```python
from build123d import *

# Parameters (mm, degrees)
SKETCH1_R           = 26
BOSS_EXTRUDE1_DEPTH = 14.2
SKETCH4_R           = 2.9
BOSS_EXTRUDE2_DEPTH = 12.7
SKETCH8_R           = 26
BOSS_EXTRUDE3_DEPTH = 25
SKETCH9_R           = 28.075
BOSS_EXTRUDE4_DEPTH = 17.2
SKETCH10_R          = 3.325
BOSS_EXTRUDE5_DEPTH = 16.45


with BuildPart() as part:
    # Sketch1 → Boss-Extrude1 (new body)
    with BuildSketch(Plane(origin=(0, 0, 0), x_dir=(1, 0, 0), z_dir=(0, 1, 0))):
        Circle(SKETCH1_R)
    extrude(amount=BOSS_EXTRUDE1_DEPTH)

    # Sketch4 → Boss-Extrude2 (add)
    with BuildSketch(Plane.XZ):
        with BuildLine():
            Line((27.12908409, -11.679561866), (37.990088974, -4.433027686))
            ThreePointArc((37.990088974, -4.433027686), (40.05, 0), (37.990088974, 4.433027686))
            Line((37.990088974, 4.433027686), (27.12908409, 11.679561866))
            ThreePointArc((27.12908409, 11.679561866), (22.194049101, 15.251075575), (17.545087541, 19.18775399))
            ThreePointArc((17.545087541, 19.18775399), (0, 26), (-17.545087541, 19.18775399))
            ThreePointArc((-17.545087541, 19.18775399), (-22.194049101, 15.251075575), (-27.12908409, 11.679561866))
            Line((-27.12908409, 11.679561866), (-37.990088974, 4.433027686))
            ThreePointArc((-37.990088974, 4.433027686), (-40.05, 0), (-37.990088974, -4.433027686))
            Line((-37.990088974, -4.433027686), (-27.12908409, -11.679561866))
            ThreePointArc((-27.12908409, -11.679561866), (-22.194049101, -15.251075575), (-17.545087541, -19.18775399))
            ThreePointArc((-17.545087541, -19.18775399), (0, -26), (17.545087541, -19.18775399))
            ThreePointArc((17.545087541, -19.18775399), (22.194049101, -15.251075575), (27.12908409, -11.679561866))
        make_face()
        with Locations((34.25, 0)):
            Circle(SKETCH4_R, mode=Mode.SUBTRACT)
        with Locations((-34.25, 0)):
            Circle(SKETCH4_R, mode=Mode.SUBTRACT)
    extrude(amount=-BOSS_EXTRUDE2_DEPTH)

    # Sketch8 → Boss-Extrude3 (add)
    with BuildSketch(Plane(origin=(0, 14.2, 0), x_dir=(1, 0, 0), z_dir=(0, 1, 0))):
        Circle(SKETCH8_R)
    extrude(amount=BOSS_EXTRUDE3_DEPTH)

    # Sketch9 → Boss-Extrude4 (add)
    with BuildSketch(Plane(origin=(0, 39.2, 0), x_dir=(1, 0, 0), z_dir=(0, 1, 0))):
        Circle(SKETCH9_R)
    extrude(amount=BOSS_EXTRUDE4_DEPTH)

    # Sketch10 → Boss-Extrude5 (add)
    with BuildSketch(Plane(origin=(0, 56.4, 0), x_dir=(1, 0, 0), z_dir=(0, 1, 0))):
        with Locations((13.3, 0)):
            Circle(SKETCH10_R)
        with Locations((-13.3, 0)):
            Circle(SKETCH10_R)
    extrude(amount=BOSS_EXTRUDE5_DEPTH)


solid = part.part
```
Here's how the part is built. I have some questions about the finished solid (model axes, mm). A direction names the side the tool comes from. Round coordinates to 2 decimals unless told otherwise and drop trailing zeros. Loops run counter-clockwise (first coordinate to the right, second up) from the corner with the lowest first, then second, coordinate; pieces in that order, holes last.
1. Suppose I cut it at C-C, the plane y = 62.5. Please give me the cut outline in (x, z) (3 decimals).
Answers:
outline: circle Ø6.65 at (-13.3, 0); circle Ø6.65 at (13.3, 0)
2. Suppose I cut it at D-D, the plane x = 0. Please give me the cut outline in (y, z) (3 decimals), and give its area (3 significant figures).
Answers:
outline: (0, -26) - (39.2, -26) - (39.2, -28.075) - (56.4, -28.075) - (56.4, 28.075) - (39.2, 28.075) - (39.2, 26) - (0, 26) - close
area: 3,000 mm2
3. If I drill on probe 1 along X at (y, z) = (5.5, -1.5); probe 2 along Y at (x, z) = (-31, -3.5); probe 3 along Y at (x, z) = (27.5, -3.5), over which ranges is the centre line in solid material (lowest first)?
Answers:
probe 1: x = -39.85 to -36.73, -31.77 to 31.77, 36.73 to 39.85
probe 2: y = 0 to 12.7
probe 3: y = 0 to 12.7, 39.2 to 56.4
4. Suppose I cut it at A-A, the plane z = 0. Please give me the cut outline in (x, y) (3 decimals), and give its area (3 significant figures).
Answers:
outline: (-40.05, 0) - (-37.15, 0) - (-37.15, 12.7) - (-40.05, 12.7) - close; (-31.35, 0) - (31.35, 0) - (31.35, 12.7) - (26, 12.7) - (26, 39.2) - (28.075, 39.2) - (28.075, 56.4) - (16.625, 56.4) - (16.625, 72.85) - (9.975, 72.85) - (9.975, 56.4) - (-9.975, 56.4) - (-9.975, 72.85) - (-16.625, 72.85) - (-16.625, 56.4) - (-28.075, 56.4) - (-28.075, 39.2) - (-26, 39.2) - (-26, 12.7) - (-31.35, 12.7) - close; (37.15, 0) - (40.05, 0) - (40.05, 12.7) - (37.15, 12.7) - close
area: 3,430 mm2
5. Suppose I cut it at B-B, the plane x = 34.25. Please give me the cut outline in (y, z).
Answers:
outline: (0, -6.93) - (12.7, -6.93) - (12.7, -2.9) - (0, -2.9) - close; (0, 2.9) - (12.7, 2.9) - (12.7, 6.93) - (0, 6.93) - close
6. Thinking about a two-plate mould opening in X: for faces 1 (the face through (16.47, 64.51, -1)), 2 (the face through (13, 72.85, 0)), 3 (the face through (-31.484, 6.261, 0.871)), 4 (the face through (26.78, 47.68, -8.43)), which applies, released by +X, released by -X, zero draft, split by the parting line, or undercut?
Answers:
face 1: undercut
face 2: zero draft
face 3: undercut
face 4: split by the parting line
7. Will these pins go through, and if not, where does the flat tip stop? pin 1 (11.5 mm diameter, centred on x = -29, z = -0.5, fed in from +Y); pin 2 (7.5 mm diameter, centred on x = -34.25, z = 0, fed in from +Y); pin 3 (5 mm diameter, centred on x = 14, y = 59.5, fed in from +Z) (3 decimals).
Answers:
pin 1: stops at y = 56.4
pin 2: stops at y = 12.7
pin 3: stops at z = 3.325
8. For faces 5 (the face through (-16.62, 64.51, -0.15)), 6 (the face through (8, 39.2, 25)), 7 (the face through (-22.26, 6.26, -15.2)), 8 (the face through (22.13, 6.26, -15.3)), which set-ups out of +Z, -Z, +X, -X, +Y, -Y let a thin tool reach every point of the face, with its end or its side?
Answers:
face 5: +Y
face 6: none
face 7: -Z, -X, -Y
face 8: -Z, +X, -Y
